Source: CAD feature listing. Evaluate the final solid. Frame: model axes, mm. A direction names the side the tool comes from. Coordinates: 2 decimals unless noted, no trailing zeros. Order: outer loops, then holes, each group sorted by start corner. A loop starts at its lowest first (then second) coordinate and runs counter-clockwise, first axis right, second up.
```python
from build123d import *

# Parameters (mm, degrees)
F0_W     = 105
F0_H     = 40
F1_DEPTH = 34
F2_W     = 96
F2_H     = 20
F3_DEPTH = 40.001
F4_W     = 96
F4_H     = 27
F5_DEPTH = 10
F6_W     = 15
F6_H     = 10
F7_DEPTH = 105.001


with BuildPart() as f1:
    # F0 (on Top) → F1 (new body)
    with BuildSketch(Plane.XY):
        with Locations((8.404606, -17.624996)):
            Rectangle(F0_W, F0_H)
    extrude(amount=F1_DEPTH)

    # F2 (on face) → F3 (cut, through all)
    with BuildSketch(Plane.XZ.offset(37.624996)):
        with Locations((8.904606, 15)):
            Rectangle(F2_W, F2_H)
    extrude(amount=-F3_DEPTH, mode=Mode.SUBTRACT)

    # F4 (on face) → F5 (cut)
    with BuildSketch(Plane.XY.offset(34)):
        with Locations((8.904606, -11.124996)):
            Rectangle(F4_W, F4_H)
    extrude(amount=-F5_DEPTH, mode=Mode.SUBTRACT)

    # F6 (on face) → F7 (cut, through all)
    with BuildSketch(Plane.YZ.offset(60.904606)):
        with Locations((-17.624996, 17)):
            Rectangle(F6_W, F6_H)
    extrude(amount=-F7_DEPTH, mode=Mode.SUBTRACT)


solid = f1.part
```
1. Draft query along X for faces 1 (the face through (-44.095, -18, 9)), 2 (the face through (8, -24.625, 30)), 3 (the face through (59, -18, 12)). Return one class per face: released by +X, released by -X, zero draft, split by the parting line, or undercut.
Findings:
face 1: released by -X
face 2: undercut
face 3: zero draft
2. Section query B-B on x = -9. Return loops of the section in (y, z) (3 decimals).
Findings:
outline: (-37.625, 0) - (2.375, 0) - (2.375, 5) - (-37.625, 5) - close; (-37.625, 25) - (-24.625, 25) - (-24.625, 34) - (-37.625, 34) - close
3. Section query C-C on z = 18. Return loops of the section in (x, y) (3 decimals), plus the area to 3 significant figures.
Findings:
outline: (-44.095, -37.625) - (-39.095, -37.625) - (-39.095, -25.125) - (-44.095, -25.125) - close; (-44.095, -10.125) - (-39.095, -10.125) - (-39.095, 2.375) - (-44.095, 2.375) - close; (56.905, -37.625) - (60.905, -37.625) - (60.905, -25.125) - (56.905, -25.125) - close; (56.905, -10.125) - (60.905, -10.125) - (60.905, 2.375) - (56.905, 2.375) - close
area: 225 mm2
4. Pin query (flat end, axial travel): P1, Ø6, axis at x = -14.5, z = 20, coming from the -Y side; P2, Ø1, axis at x = -6.5, y = -18.5, coming from the +Z side; P3, Ø10, axis at x = -9, z = 31.5, coming from the +Y side (3 decimals). Return the tip coordinate at first contact, or that it passes through.
Findings:
P1: passes through
P2: stops at z = 5
P3: stops at y = -24.625
5. Ray query, line 1 (Z direction, x = -26, y = -26.5); line 2 (X direction, y = -6, z = 21); line 3 (Y direction, x = 39, z = 27.5) (3 decimals). Return the intervals inside material, ascending.
Findings:
line 1: z = 0 to 5, 25 to 34
line 2: x = -44.1 to -39.1, 56.9 to 60.9
line 3: y = -37.625 to -24.625
6. Section query D-D on y = -26.5. Return loops of the section in (x, z).
Findings:
outline: (-44.1, 0) - (60.9, 0) - (60.9, 34) - (-44.1, 34) - close; hole (-39.1, 5) - (56.9, 5) - (56.9, 25) - (-39.1, 25) - close
7. Section query A-A on z = 11. Return loops of the section in (x, y) (3 decimals).
Findings:
outline: (-44.095, -37.625) - (-39.095, -37.625) - (-39.095, 2.375) - (-44.095, 2.375) - close; (56.905, -37.625) - (60.905, -37.625) - (60.905, 2.375) - (56.905, 2.375) - close
8. Access query for faces 4 (the face through (56.905, -18, 23)), 5 (the face through (-42, -18, 22)), 6 (the face through (8, -31, 25)), 7 (the face through (8, -17, 0)). Directions: +Z, -Z, +X, -X, +Y, -Y. A direction counts if a zero-diameter tool reaches every point of the face in a straight line with its end or side. Return the directions, or none.
Findings:
face 4: +Y
face 5: +X, -X
face 6: +Y, -Y
face 7: -Z, +X, -X, +Y, -Y
